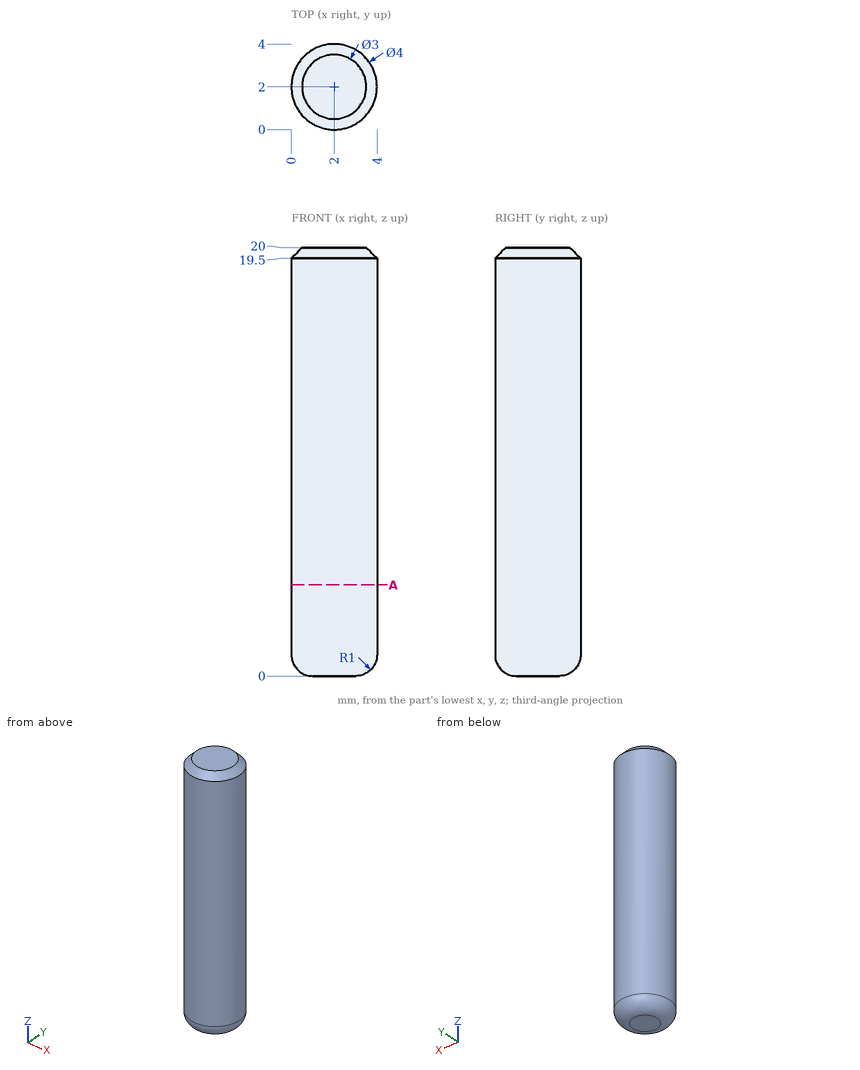
The drawing under review shows one solid part. Ordinate dimensions are in mm from its lowest x, y, z. Round coordinates to 2 decimals unless told otherwise and drop trailing zeros. Loops run counter-clockwise (first coordinate to the right, second up) from the corner with the lowest first, then second, coordinate; pieces in that order, holes last. Notation, with made-up numbers: (-8.5, 0.25) -> (20.5, 0.25) arc R23 ccw to (20.5, 22.25) -> close; hole circle Ø7 at (-10, 31). An arc over 180 degrees is marked (long way). One line per question, with ' | ' between items. Start each with the question number.
Item 1: Add section A-A, the plane z = 4.25. Write out the cut boundary in (x, y), then the cut area to 3 significant figures.
Item 2: Wall thickness on line 1 along X through (y, z) = (1.9, 6); line 2 along Y through (x, z) = (2.2, 4.25); line 3 along Z through (x, y) = (2.8, 1): over which ranges is each line inside the solid? List them lowest first. Write a range as [from, to].
Item 3: For pin 1 (2 mm diameter, centred on y = 3.5, z = 4, fed in from -X), flat-tipped, find the tip position at first contact; note if it passes through.
Return value:
1) outline: circle Ø4 at (2, 2) | area: 12.6 mm2
2) line 1: x = [0, 4] | line 2: y = [0.01, 3.99] | line 3: z = [0.04, 20]
3) pin 1: stops at x = 0.06
